Job drawing, mm, ordinate dimensions from the low corner. One solid piece. A direction names the side the tool comes from. Round coordinates to 2 decimals unless told otherwise and drop trailing zeros. Order: outer loops, then holes, each group sorted by start corner. A loop starts at its lowest first (then second) coordinate and runs counter-clockwise, first axis right, second up. Notation, with made-up numbers: (70, 49) -> (85, 49) arc R20 cw to (85, 83) -> close; hole circle Ø5 at (24, -33.75). An arc over 180 degrees is marked (long way). Use CSV: the item, a comma, the result in double quotes.
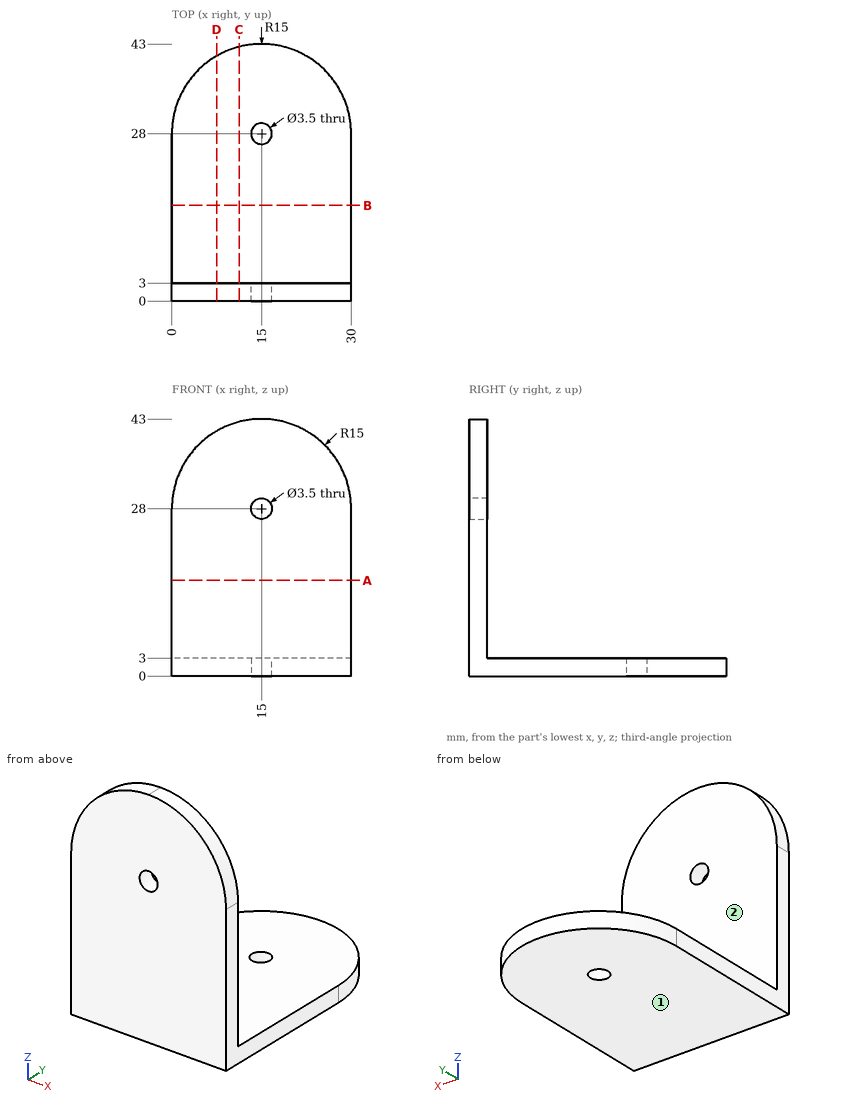
(1) Which spindle directions (+Z, -Z, +X, -X, +Y, -Y) get a long thin tool onto all of the face, cutting with end or side? Do the marked faces 1 and 2. Say none if no direction does.
Reply:
face 1,"-Z, +X, -X, +Y, -Y"
face 2,"+Z, +X, -X, +Y"
(2) Probe probe 1 along X at (y, z) = (2, 28); probe 2 along Y at (x, z) = (15, 2.2); probe 3 along Y at (x, z) = (6, 17). List the from-to ranges inside material, lowest first. Write a range as [from, to].
Reply:
probe 1,"[0, 13.25], [16.75, 30]"
probe 2,"[0, 26.25], [29.75, 43]"
probe 3,"[0, 3]"
(3) Cut at C-C, the plane x = 11.25. Give the cut face in (y, z), then the cut area to 3 significant figures.
Reply:
outline,"(0, 0) -> (42.52, 0) -> (42.52, 3) -> (3, 3) -> (3, 42.52) -> (0, 42.52) -> close"
area,"246 mm2"
(4) Drop flat-ended pins along their axis: P1, Ø1.5, axis at x = 21.5, z = 13.5, coming from the -Y side; P2, Ø10, axis at y = 9, z = 32.5, coming from the +X side; P3, Ø15, axis at x = 15, y = 16.5, coming from the +Z side; P4, Ø15, axis at x = 18, z = 23, coming from the +Y side. Give the stop position or say it passes through.
Reply:
P1,"y = 0"
P2,"through"
P3,"z = 3"
P4,"y = 3"
(5) Cut at A-A, the plane z = 16. Give the cut face in (x, y).
Reply:
outline,"(0, 0) -> (30, 0) -> (30, 3) -> (0, 3) -> close"
(6) Cut at D-D, the plane x = 7.5. Give the cut face in (y, z), then the cut area to 3 significant figures.
Reply:
outline,"(0, 0) -> (40.99, 0) -> (40.99, 3) -> (3, 3) -> (3, 40.99) -> (0, 40.99) -> close"
area,"237 mm2"
